```python
from build123d import *

# Parameters (mm, degrees)
SKETCH_1_W                     = 80
SKETCH_1_H                     = 60
EXTRUDE_1_DEPTH                = 8
HOLE_WIZARD_M3_5_1_D           = 4
HOLE_WIZARD_M3_5_1_CBORE_D     = 8
HOLE_WIZARD_M3_5_1_CBORE_DEPTH = 2
SKETCH_14_W                    = 80
SKETCH_14_H                    = 2
SKETCH_14_W_2                  = 2
SKETCH_14_H_2                  = 16
CUT_EXTRUDE_1_DEPTH            = 1
CUT_EXTRUDE_2_REACH            = 92.174
SKETCH_15_R                    = 4.25
SKETCH_17_R                    = 11.5
CUT_EXTRUDE_4_DEPTH            = 4
SKETCH_18_R                    = 6
CUT_EXTRUDE_5_DEPTH            = 3
CHAMFER_1_SIZE                 = 1.499999999
CHAMFER_1_SIZE2                = 1.500000001
CHAMFER_2_SIZE                 = 1
SKETCH_20_W                    = 80
SKETCH_20_H                    = 6
CUT_EXTRUDE_6_DEPTH            = 1
SKETCH_21_W                    = 80
SKETCH_21_H                    = 4
CUT_EXTRUDE_7_DEPTH            = 1
SKETCH_22_W                    = 80
SKETCH_22_H                    = 2
CUT_EXTRUDE_8_DEPTH            = 1
SKETCH_23_R                    = 1
CUT_EXTRUDE_9_DEPTH            = 1
CUT_EXTRUDE_10_REACH           = 92.174
SKETCH_24_W                    = 80
SKETCH_24_H                    = 20
EXTRUDE_2_DEPTH                = 3
CUT_EXTRUDE_11_REACH           = 92.174


with BuildPart() as part:
    # 草图1 → 凸台-拉伸1 (new body)
    with BuildSketch(Plane.XY.offset(8)):
        with Locations((40, 10.833333333)):
            Rectangle(SKETCH_1_W, SKETCH_1_H)
    extrude(amount=-EXTRUDE_1_DEPTH)

    # M3.5 六角头机械螺钉的柱形沉头孔1 (through all)
    with Locations(Plane.XY.offset(8)):
        with Locations((8, 15.833333333), (72, 15.833333333)):
            CounterBoreHole(HOLE_WIZARD_M3_5_1_D / 2, HOLE_WIZARD_M3_5_1_CBORE_D / 2, HOLE_WIZARD_M3_5_1_CBORE_DEPTH)

    # 草图14 → 切除-拉伸1 (cut)
    with BuildSketch(Plane.XY.offset(8)):
        with Locations((40, 37.833333333)):
            Rectangle(SKETCH_14_W, SKETCH_14_H)
        Polygon((15, 40.833333333), (31, 24.833333333), (32.414213562, 26.247546896), (16.414213562, 42.247546896), align=None)
        with Locations((7, 32.833333333)):
            Rectangle(SKETCH_14_W_2, SKETCH_14_H_2)
        with Locations((40, 32.833333333)):
            Rectangle(SKETCH_14_W_2, SKETCH_14_H_2)
        with Locations((73, 32.833333333)):
            Rectangle(SKETCH_14_W_2, SKETCH_14_H_2)
        Polygon((47.585786438, 26.247546896), (63.585786438, 42.247546896), (65, 40.833333333), (49, 24.833333333), align=None)
    extrude(amount=-CUT_EXTRUDE_1_DEPTH, mode=Mode.SUBTRACT)

    # 草图15 → 切除-拉伸2 (cut, up to next)
    with BuildSketch(Plane.XY.offset(8), mode=Mode.PRIVATE) as cut_extrude_2_sk1:
        with Locations((40, 15.833333333)):
            Circle(SKETCH_15_R)
    cut_extrude_2_tool1 = extrude(cut_extrude_2_sk1.sketch, amount=-CUT_EXTRUDE_2_REACH, mode=Mode.PRIVATE) & part.part
    add(cut_extrude_2_tool1.solids().sort_by_distance((40, 15.833333, 8))[0], mode=Mode.SUBTRACT)

    # 草图17 → 切除-拉伸4 (cut)
    with BuildSketch(Plane.XY.offset(8)):
        with Locations((40, 15.833333333)):
            Circle(SKETCH_17_R)
    extrude(amount=-CUT_EXTRUDE_4_DEPTH, mode=Mode.SUBTRACT)

    # 草图18 → 切除-拉伸5 (cut)
    with BuildSketch(Plane(origin=(0, 0, 0), x_dir=(-1, 0, 0), z_dir=(0, 0, -1))):
        with Locations((-40, 15.833333333)):
            Circle(SKETCH_18_R)
    extrude(amount=-CUT_EXTRUDE_5_DEPTH, mode=Mode.SUBTRACT)

    # 倒角1
    chamfer_1_edges = [part.edges().sort_by_distance(p)[0] for p in [
        (74, 15.833333333, 0),
        (10, 15.833333333, 0),
    ]]
    chamfer_1_side = [part.faces().sort_by_distance(p)[0] for p in [
        (79, 10.833333333, 0),
    ]]
    chamfer(chamfer_1_edges, length=CHAMFER_1_SIZE, length2=CHAMFER_1_SIZE2, reference=chamfer_1_side[0])

    # 倒角2
    chamfer_2_edges = [part.edges().sort_by_distance(p)[0] for p in [
        (40, 40.833333333, 0),
    ]]
    chamfer(chamfer_2_edges, length=CHAMFER_2_SIZE)

    # 草图20 → 切除-拉伸6 (cut)
    with BuildSketch(Plane.XY.offset(8)):
        with Locations((40, -16.166666667)):
            Rectangle(SKETCH_20_W, SKETCH_20_H)
    extrude(amount=-CUT_EXTRUDE_6_DEPTH, mode=Mode.SUBTRACT)

    # 草图21 → 切除-拉伸7 (cut)
    with BuildSketch(Plane.XY.offset(7)):
        with Locations((40, -17.166666667)):
            Rectangle(SKETCH_21_W, SKETCH_21_H)
    extrude(amount=-CUT_EXTRUDE_7_DEPTH, mode=Mode.SUBTRACT)

    # 草图22 → 切除-拉伸8 (cut)
    with BuildSketch(Plane.XY.offset(6)):
        with Locations((40, -18.166666667)):
            Rectangle(SKETCH_22_W, SKETCH_22_H)
    extrude(amount=-CUT_EXTRUDE_8_DEPTH, mode=Mode.SUBTRACT)

    # 草图23 → 切除-拉伸9 (cut)
    with BuildSketch(Plane.XY.offset(8)):
        with Locations((7, 24.833333333)):
            Circle(SKETCH_23_R)
        with Locations((31.707106781, 25.540440115)):
            Circle(SKETCH_23_R)
        with Locations((48.292893219, 25.540440115)):
            Circle(SKETCH_23_R)
        with Locations((73, 24.833333333)):
            Circle(SKETCH_23_R)
    extrude(amount=-CUT_EXTRUDE_9_DEPTH, mode=Mode.SUBTRACT)

    # 草图24 → 切除-拉伸10 (cut, up to next)
    with BuildSketch(Plane.XY.offset(8), mode=Mode.PRIVATE) as cut_extrude_10_sk1:
        with Locations((40, -9.166666667)):
            Rectangle(SKETCH_24_W, SKETCH_24_H)
    cut_extrude_10_tool1 = extrude(cut_extrude_10_sk1.sketch, amount=-CUT_EXTRUDE_10_REACH, mode=Mode.PRIVATE) & part.part
    add(cut_extrude_10_tool1.solids().sort_by_distance((40, -9.166667, 8))[0], mode=Mode.SUBTRACT)

    # 草图25 → 凸台-拉伸2 (add)
    with BuildSketch(Plane.XY.offset(8)):
        with BuildLine():
            Line((0, 40.833333333), (80, 40.833333333))
            Line((80, 40.833333333), (80, 22.833333333))
            Line((80, 22.833333333), (49.124143795, 22.833333333))
            ThreePointArc((49.124143795, 22.833333333), (40, 27.333333333), (30.875856205, 22.833333333))
            Line((30.875856205, 22.833333333), (0, 22.833333333))
            Line((0, 22.833333333), (0, 40.833333333))
        make_face()
    extrude(amount=-EXTRUDE_2_DEPTH)

    # 草图26 → 切除-拉伸11 (cut, up to next)
    with BuildSketch(Plane.ZY, mode=Mode.PRIVATE) as cut_extrude_11_sk1:
        Polygon((4.8, 40.833333333), (4.8, 40.033333333), (5.6, 40.033333333), (5.6, 39.233333333), (6.4, 39.233333333), (6.4, 38.433333333), (7.2, 38.433333333), (7.2, 37.633333333), (8, 37.633333333), (8, 40.833333333), align=None)
    cut_extrude_11_tool1 = extrude(cut_extrude_11_sk1.sketch, amount=-CUT_EXTRUDE_11_REACH, mode=Mode.PRIVATE) & part.part
    add(cut_extrude_11_tool1.solids().sort_by_distance((0, 39.633333, 6.8))[0], mode=Mode.SUBTRACT)


solid = part.part
```
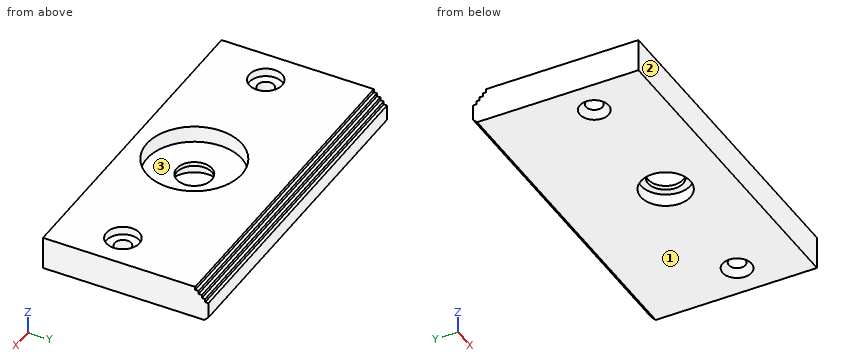
Read the model definition and answer for the solid it produces. Units are mm, in the model's axes. Face numbers are marked on the shaded views. Round coordinates to 2 decimals unless told otherwise and drop trailing zeros. Write each loop counter-clockwise with the first axis right and the second up, starting at its lowest first coordinate (ties: lowest second). Pieces come first, ordered by that corner, then holes. Notation, with made-up numbers: (36, 30) - (95, 30) arc R22 cw to (95, 51) - close; hole circle Ø7 at (85.25, -18.5). An arc over 180 degrees is marked (long way). One line per item, written item: value.
Q1. Find section C-C (y = 25.5). Determine the outline of the cut face in (x, z), and give its area (3 significant figures).
The answers:
outline: (0, 0) - (80, 0) - (80, 8) - (46.23, 8) - (46.23, 4) - (33.77, 4) - (33.77, 8) - (0, 8) - close
area: 590 mm2
Q2. Each of these flat-tipped pins is pushed along its axis until it touches: P1, Ø3.5, axis at x = 40.5, y = 15, coming from the -Z side; P2, Ø0.6, axis at x = 37.5, z = 7, coming from the +Y side; P3, Ø4, axis at x = 6.5, y = 16.5, coming from the +Z side; P4, Ø0.6, axis at x = 36, z = 6, coming from the +Y side. Where does it stop, or does it pass through?
The answers:
P1: passes through
P2: stops at y = 38.43
P3: stops at z = 6
P4: stops at y = 39.23
Q3. Find section A-A (x = 40). Determine the outline of the cut face in (y, z), and give its area (3 significant figures).
The answers:
outline: (0.83, 0) - (9.83, 0) - (9.83, 3) - (11.58, 3) - (11.58, 4) - (4.33, 4) - (4.33, 8) - (0.83, 8) - close; (20.08, 3) - (21.83, 3) - (21.83, 0) - (39.83, 0) - (40.83, 1) - (40.83, 4.8) - (40.03, 4.8) - (40.03, 5.6) - (39.23, 5.6) - (39.23, 6.4) - (38.43, 6.4) - (38.43, 7.2) - (37.63, 7.2) - (37.63, 8) - (27.33, 8) - (27.33, 4) - (20.08, 4) - close
area: 177 mm2
Q4. For a pull along Y with two mould halves and no side action, classify the marked faces 1, 2 and 3 as pulls with the +Y half, pulls with the -Y half, needs draft (parallel to the pull), parting line crosses it, or undercut.
The answers:
face 1: needs draft
face 2: pulls with the -Y half
face 3: undercut
Q5. Find section B-B (x = 14). Determine the outline of the cut face in (y, z), and give its area (3 significant figures).
The answers:
outline: (0.83, 0) - (39.83, 0) - (40.83, 1) - (40.83, 4.8) - (40.03, 4.8) - (40.03, 5.6) - (39.23, 5.6) - (39.23, 6.4) - (38.43, 6.4) - (38.43, 7.2) - (37.63, 7.2) - (37.63, 8) - (0.83, 8) - close
area: 313 mm2
Q6. Straight lines are drawn through the part: line 1 (Y direction, x = 8, z = 4.35); line 2 (Y direction, x = 40, z = 3.5); line 3 (X direction, y = 14, z = 7.75). For each, find the intervals that lie inside material, in ascending order. Write a range as from..to.
The answers:
line 1: y = 0.83..13.83, 17.83..40.83
line 2: y = 0.83..11.58, 20.08..40.83
line 3: x = 0..4.44, 11.56..28.65, 51.35..68.44, 75.56..80
